from build123d import *

# Parameters (mm, degrees)
SKETCH1_W           = 10
SKETCH1_H           = 55
SKETCH1_W_2         = 4.5
SKETCH1_H_2         = 4
SKETCH1_H_3         = 2
BOSS_EXTRUDE2_DEPTH = 5
SKETCH2_W           = 5
SKETCH2_H           = 10
SKETCH2_W_2         = 10
CUT_EXTRUDE1_DEPTH  = 2
CUT_EXTRUDE2_DEPTH  = 30.223335826
SKETCH4_W           = 3
SKETCH4_H           = 2
CUT_EXTRUDE3_DEPTH  = 1.5
CUT_EXTRUDE4_DEPTH  = 3


with BuildPart() as part:
    # Sketch1 → Boss-Extrude2 (new body)
    # profile 1 of 3: a face of its own
    with BuildSketch(Plane.XY.offset(13.5)):
        with Locations((-4.4209, 0)):
            Rectangle(SKETCH1_W, SKETCH1_H)
        with Locations((-4.4209, 0)):
            Rectangle(SKETCH1_W_2, SKETCH1_H_2, mode=Mode.SUBTRACT)
    # profile 2 of 3: a face of its own
    with BuildSketch(Plane.XY.offset(13.5)):
        with Locations((-4.4209, -1)):
            Rectangle(SKETCH1_W_2, SKETCH1_H_3)
    # profile 3 of 3: a face of its own
    with BuildSketch(Plane.XY.offset(13.5)):
        with Locations((-4.4209, 1)):
            Rectangle(SKETCH1_W_2, SKETCH1_H_3)
    extrude(amount=BOSS_EXTRUDE2_DEPTH)

    # Sketch2 → Cut-Extrude1 (cut)
    with BuildSketch(Plane.XY.offset(18.5)):
        with Locations((-6.9209, 22.5)):
            Rectangle(SKETCH2_W, SKETCH2_H)
        with Locations((-1.9209, 22.5)):
            Rectangle(SKETCH2_W, SKETCH2_H)
        with Locations((-4.4209, -22.5)):
            Rectangle(SKETCH2_W_2, SKETCH2_H)
    extrude(amount=-CUT_EXTRUDE1_DEPTH, mode=Mode.SUBTRACT)

    # Sketch3 → Cut-Extrude2 (cut, through all)
    with BuildSketch(Plane.XY.offset(16.5)):
        with BuildLine():
            ThreePointArc((-2.5209, 22.5), (-3.077397116, 23.843502884), (-4.4209, 24.4))
            Line((-4.4209, 24.4), (-4.4209, 20.6))
            ThreePointArc((-4.4209, 20.6), (-3.077397116, 21.156497116), (-2.5209, 22.5))
        make_face()
        with BuildLine():
            Line((-4.4209, 20.6), (-4.4209, 24.4))
            ThreePointArc((-4.4209, 24.4), (-6.3209, 22.5), (-4.4209, 20.6))
        make_face()
        with BuildLine():
            ThreePointArc((-2.5209, -22.5), (-3.077397116, -21.156497116), (-4.4209, -20.6))
            Line((-4.4209, -20.6), (-4.4209, -24.4))
            ThreePointArc((-4.4209, -24.4), (-3.077397116, -23.843502884), (-2.5209, -22.5))
        make_face()
        with BuildLine():
            Line((-4.4209, -24.4), (-4.4209, -20.6))
            ThreePointArc((-4.4209, -20.6), (-6.3209, -22.5), (-4.4209, -24.4))
        make_face()
    extrude(amount=-CUT_EXTRUDE2_DEPTH, mode=Mode.SUBTRACT)

    # Sketch4 → Cut-Extrude3 (cut)
    with BuildSketch(Plane(origin=(0, 0, 13.5), x_dir=(-1, 0, 0), z_dir=(0, 0, -1))):
        with Locations((4.4209, -1)):
            Rectangle(SKETCH4_W, SKETCH4_H)
        with Locations((4.4209, 1)):
            Rectangle(SKETCH4_W, SKETCH4_H)
    extrude(amount=-CUT_EXTRUDE3_DEPTH, mode=Mode.SUBTRACT)

    # Sketch5 → Cut-Extrude4 (cut)
    with BuildSketch(Plane.ZY.offset(2.9209)):
        Polygon((18.5, 7), (18.5, 5.5), (15, 2), (13.5, 2), align=None)
    extrude(amount=CUT_EXTRUDE4_DEPTH, mode=Mode.SUBTRACT)


solid = part.part
Source: CAD feature listing. Evaluate the final solid. Frame: model axes, mm. A direction names the side the tool comes from. Give positions to 0.01 mm unless a question says otherwise; leave off trailing zeros. Write each loop counter-clockwise with the first axis right and the second up, starting at its lowest first coordinate (ties: lowest second). Pieces come first, ordered by that corner, then holes. Notation, with made-up numbers: M 47,-28 L 94,-28 A14 cw 94,-1 Z; hole C 3,17.5 d7. An arc over 180 degrees is marked long. Answer as a JSON object with one key per item and string values.
Q1. Ray query, line 1 along Z through (x, y) = (-0.75, -20); line 2 along Y through (x, z) = (-4.75, 18.1); line 3 along X through (y, z) = (-22, 15.85). Return the intervals inside material, ascending.
Geometry check:
{"line 1": "z = 13.5 to 16.5", "line 2": "y = -17.5 to 5.1, 6.6 to 17.5", "line 3": "x = -9.42 to -6.25, -2.59 to 0.58"}
Q2. Cut plane D-D, the plane x = -8. Return the cut outline in (y, z), then the cut area to 3 significant figures.
Geometry check:
{"outline": "M -27.5,13.5 L 27.5,13.5 L 27.5,16.5 L 17.5,16.5 L 17.5,18.5 L -17.5,18.5 L -17.5,16.5 L -27.5,16.5 Z", "area": "235 mm^2"}
Q3. Cut plane A-A, the plane z = 17.85. Return the cut outline in (x, y), then the cut area to 4 significant figures.
Geometry check:
{"outline": "M -9.42,-17.5 L 0.58,-17.5 L 0.58,17.5 L -9.42,17.5 Z; hole M -5.92,4.85 L -2.92,4.85 L -2.92,6.35 L -5.92,6.35 Z", "area": "345.5 mm^2"}
Q4. Access query for faces 4 (the face through (-4, 17.5, 18)), 5 (the face through (-5.921, 2.5, 15.2)), 6 (the face through (-4, 0, 18.5)), 7 (the face through (-4, -17.5, 18)), 8 (the face through (-4, -2, 14)). Directions: +Z, -Z, +X, -X, +Y, -Y. A direction counts if a zero-diameter tool reaches every point of the face in a straight line with its end or side. Return the directions, or none.
Geometry check:
{"face 4": "+Z, +X, -X, +Y", "face 5": "none", "face 6": "+Z, +X, -X, +Y, -Y", "face 7": "+Z, +X, -X, -Y", "face 8": "-Z"}
Q5. Cut plane B-B, the plane y = -23.5. Return the cut outline in (x, z), then the cut area to 3 significant figures.
Geometry check:
{"outline": "M -9.42,13.5 L -6.04,13.5 L -6.04,16.5 L -9.42,16.5 Z; M -2.81,13.5 L 0.58,13.5 L 0.58,16.5 L -2.81,16.5 Z", "area": "20.3 mm^2"}
Q6. Contact query for flat-ended pins moving along their axis: P1, Ø3, axis at x = -3.5, y = 21, coming from the +Z side; P2, Ø1.5, axis at x = -5, z = 17.5, coming from the -Y side; P3, Ø2, axis at x = -4, z = 18, coming from the +Y side. Output: stop coordinate, or through.
Geometry check:
{"P1": "stops at z = 16.5", "P2": "stops at y = -17.5", "P3": "stops at y = 17.5"}
Q7. Cut plane C-C, the plane x = -5. Return the cut outline in (y, z), then the cut area to 3 significant figures.
Geometry check:
{"outline": "M -27.5,13.5 L -24.31,13.5 L -24.31,16.5 L -27.5,16.5 Z; M -20.69,13.5 L -2,13.5 L -2,15 L 2,15 L 5.5,18.5 L -17.5,18.5 L -17.5,16.5 L -20.69,16.5 Z; M 2,13.5 L 20.69,13.5 L 20.69,16.5 L 17.5,16.5 L 17.5,18.5 L 7,18.5 Z; M 24.31,13.5 L 27.5,13.5 L 27.5,16.5 L 24.31,16.5 Z", "area": "201 mm^2"}
Q8. Mould query, pull axis Z, two halves, no side actions, for faces 1 (the face through (-4.4, 4.5, 16)), 2 (the face through (0.579, 0, 15)), 3 (the face through (-2, 23, 16.5)). Classes: +Z half, -Z half, draft (parallel to the pull), parting line (faces both ways), or undercut.
Geometry check:
{"face 1": "undercut", "face 2": "draft", "face 3": "+Z half"}
